Design review of the part built by this model. Coordinates are the model's own, in mm. A direction names the side the tool comes from. Round coordinates to 2 decimals unless told otherwise and drop trailing zeros. Loops run counter-clockwise (first coordinate to the right, second up) from the corner with the lowest first, then second, coordinate; pieces in that order, holes last. Notation, with made-up numbers: M 21,39.25 L 46,39.25 A13 ccw 46,57.25 Z; hole C -21,87.25 d11. An arc over 180 degrees is marked long. Use a Markdown table: item, result.
from build123d import *

# Parameters (mm, degrees)
F0_W      = 203.2
F0_H      = 203.2
F1_DEPTH  = 203.2
F2_R      = 25.4
F3_W      = 50.8
F3_H      = 50.8
F4_DEPTH  = 12.7
F5_W      = 50.8
F5_H      = 50.8
F6_DEPTH  = 12.7
F12_DEPTH = 177.8


# Not quite as in the source:
# - a feature of the source that left no trace in its solid (it failed there, or was rolled back) is left out


with BuildPart() as f1:
    # F0 (on Top) → F1 (new body)
    with BuildSketch(Plane.XY):
        Rectangle(F0_W, F0_H)
    extrude(amount=F1_DEPTH)

    # F2
    f2_edges = [f1.edges().sort_by_distance(p)[0] for p in [
        (0, 101.6, 203.2),
        (-101.6, 0, 203.2),
        (0, -101.6, 203.2),
        (101.6, 0, 203.2),
        (-101.6, -101.6, 101.6),
        (101.6, -101.6, 101.6),
        (0, -101.6, 0),
        (-101.6, 101.6, 101.6),
        (-101.6, 0, 0),
        (101.6, 101.6, 101.6),
        (0, 101.6, 0),
        (101.6, 0, 0),
    ]]
    fillet(f2_edges, radius=F2_R)

    # F3 (on face) → F4 (cut)
    with BuildSketch(Plane.XY.offset(203.2)):
        with BuildLine():
            Line((50.8, 76.2), (-50.8, 76.2))
            ThreePointArc((-50.8, 76.2), (-68.7605122421, 68.7605122421), (-76.2, 50.8))
            Line((-76.2, 50.8), (-76.2, -50.8))
            ThreePointArc((-76.2, -50.8), (-68.7605122421, -68.7605122421), (-50.8, -76.2))
            Line((-50.8, -76.2), (50.8, -76.2))
            ThreePointArc((50.8, -76.2), (68.7605122421, -68.7605122421), (76.2, -50.8))
            Line((76.2, -50.8), (76.2, 50.8))
            ThreePointArc((76.2, 50.8), (68.7605122421, 68.7605122421), (50.8, 76.2))
        make_face()
        Rectangle(F3_W, F3_H, mode=Mode.SUBTRACT)
    extrude(amount=-F4_DEPTH, mode=Mode.SUBTRACT)

    # F5 (on face) → F6 (cut)
    with BuildSketch(Plane.XY.offset(203.2)):
        with BuildLine():
            Line((-25.4, 25.4), (25.4, 25.4))
            ThreePointArc((25.4, 25.4), (0, 35.9210244843), (-25.4, 25.4))
        make_face()
        with BuildLine():
            Line((-25.4, -25.4), (-25.4, 25.4))
            ThreePointArc((-25.4, 25.4), (-35.9210244843, 0), (-25.4, -25.4))
        make_face()
        with BuildLine():
            ThreePointArc((-25.4, -25.4), (0, -35.9210244843), (25.4, -25.4))
            Line((25.4, -25.4), (-25.4, -25.4))
        make_face()
        Rectangle(F5_W, F5_H)
        with BuildLine():
            ThreePointArc((25.4, -25.4), (33.1866993079, -13.7463809437), (35.9210244843, 0))
            ThreePointArc((35.9210244843, 0), (33.1866993079, 13.7463809437), (25.4, 25.4))
            Line((25.4, 25.4), (25.4, -25.4))
        make_face()
    extrude(amount=-F6_DEPTH, mode=Mode.SUBTRACT)

    # F11 (on offset) → F12 (cut)
    with BuildSketch(Plane.XY.offset(228.6)):
        with BuildLine():
            Line((50.8, 76.2), (-50.8, 76.2))
            ThreePointArc((-50.8, 76.2), (-68.7605122421, 68.7605122421), (-76.2, 50.8))
            Line((-76.2, 50.8), (-76.2, -50.8))
            ThreePointArc((-76.2, -50.8), (-68.7605122421, -68.7605122421), (-50.8, -76.2))
            Line((-50.8, -76.2), (50.8, -76.2))
            ThreePointArc((50.8, -76.2), (68.7605122421, -68.7605122421), (76.2, -50.8))
            Line((76.2, -50.8), (76.2, 50.8))
            ThreePointArc((76.2, 50.8), (68.7605122421, 68.7605122421), (50.8, 76.2))
        make_face()
    extrude(amount=-F12_DEPTH, mode=Mode.SUBTRACT)


solid = f1.part
1. Take a section at B-B on x = -21. Give the boundary of the cut face in (y, z), and give its area (3 significant figures).
Check values:
| item | result |
|---|---|
| outline | M -101.6,25.4 A25.4 ccw -76.2,0 L 76.2,0 A25.4 ccw 101.6,25.4 L 101.6,177.8 A25.4 ccw 76.2,203.2 L 76.2,50.8 L -76.2,50.8 L -76.2,203.2 A25.4 ccw -101.6,177.8 Z |
| area | 17,500 mm² |
2. Wall thickness on line 1 along X through (y, z) = (-36, 144); line 2 along Z through (x, y) = (7.5, -34): over which ranges is each line inside the solid? List them lowest first. Write a range as from..to.
Check values:
| item | result |
|---|---|
| line 1 | x = -101.6..-76.2, 76.2..101.6 |
| line 2 | z = 0..50.8 |
3. Take a section at D-D on z = 18. Give the boundary of the cut face in (x, y), and give its area (3 significant figures).
Check values:
| item | result |
|---|---|
| outline | M -100.5,-76.2 A24.3 ccw -76.2,-100.5 L 76.2,-100.5 A24.3 ccw 100.5,-76.2 L 100.5,76.2 A24.3 ccw 76.2,100.5 L -76.2,100.5 A24.3 ccw -100.5,76.2 Z |
| area | 39,900 mm² |
4. Take a section at C-C on y = -65. Give the boundary of the cut face in (x, z), and give its area (3 significant figures).
Check values:
| item | result |
|---|---|
| outline | M -101.6,25.4 A25.4 ccw -76.2,0 L 76.2,0 A25.4 ccw 101.6,25.4 L 101.6,177.8 A25.4 ccw 76.2,203.2 L 71.86,203.2 L 71.86,50.8 L -71.86,50.8 L -71.86,203.2 L -76.2,203.2 A25.4 ccw -101.6,177.8 Z |
| area | 18,800 mm² |
5. Machinability: for faces 5 (the face through (-1, 1, 50.8)), 6 (the face through (-71, -70, 203.2)), which of the approach directions +Z, -Z, +X, -X, +Y, -Y give a long, thin tool a straight path to every point of the face, cutting with its end or side? Answer none if there is none.
Check values:
| item | result |
|---|---|
| face 5 | +Z |
| face 6 | +Z, +X, -X, +Y, -Y |
6. Insertion check: pin 1 (1.5 mm diameter, centred on x = -3, y = -75, fed in from +Z); pin 2 (1.5 mm diameter, centred on x = 35.5, y = 72, fed in from -Z); pin 3 (8 mm diameter, centred on x = -81, z = 33.5, fed in from +Y). Each pin has a flat end and moves straight along its axis. Give the tip position at first contact, or say it passes through.
Check values:
| item | result |
|---|---|
| pin 1 | stops at z = 50.8 |
| pin 2 | stops at z = 0 |
| pin 3 | stops at y = 101.59 |
7. Take a section at A-A on z = 141. Give the boundary of the cut face in (x, y).
Check values:
| item | result |
|---|---|
| outline | M -101.6,-76.2 A25.4 ccw -76.2,-101.6 L 76.2,-101.6 A25.4 ccw 101.6,-76.2 L 101.6,76.2 A25.4 ccw 76.2,101.6 L -76.2,101.6 A25.4 ccw -101.6,76.2 Z; hole M -76.2,-50.8 A25.4 ccw -50.8,-76.2 L 50.8,-76.2 A25.4 ccw 76.2,-50.8 L 76.2,50.8 A25.4 ccw 50.8,76.2 L -50.8,76.2 A25.4 ccw -76.2,50.8 Z |
8. The part is to be moulded in two halves that separate along X. For faces 1 (the face through (68.56, -68.96, 128.07)), 2 (the face through (101.6, -1, 101)), 3 (the face through (-94.36, 1.07, 195.56)), 4 (the face through (68.96, 68.56, 128.07)), say which applies: pulls with the +X half, pulls with the -X half, needs draft (parallel to the pull), parting line crosses it, or undercut.
Check values:
| item | result |
|---|---|
| face 1 | undercut |
| face 2 | pulls with the +X half |
| face 3 | pulls with the -X half |
| face 4 | undercut |
